```python
from build123d import *

# Parameters (mm, degrees)
REVOLVE_1_ANGLE = 359


with BuildPart() as part:
    # 草图2 → 旋转1 (revolve)
    with BuildSketch(Plane(origin=(0, 0, 0), x_dir=(0, 1, 0), z_dir=(-1, 0, 0))):
        Polygon((37, 0), (41, 0), (41, 0.5), (40.5, 0.5), (40.5, 1), (38.5, 1), (38.5, 2), (40.5, 2), (40.5, 2.5), (41, 2.5), (41, 3), (37, 3), align=None)
    revolve(axis=Axis((0, 0, 0), (0, 0, -1)), revolution_arc=REVOLVE_1_ANGLE)


solid = part.part
```
Geometry check sheet. Reference: the model listing, model coordinates, mm. A direction names the side the tool comes from. Give positions to 0.01 mm unless a question says otherwise; leave off trailing zeros. Loops run counter-clockwise (first coordinate to the right, second up) from the corner with the lowest first, then second, coordinate; pieces in that order, holes last. Notation, with made-up numbers: M 50,56.25 L 59,56.25 A10 cw 59,71.25 Z; hole C 49,34.5 d2. An arc over 180 degrees is marked long. Write item = value, one per line.
(1) Sectioned sample at A-A, the plane y = 0. Record the cut outline in (x, z).
Answer below:
outline = M -41,-3 L -37,-3 L -37,0 L -41,0 L -41,-0.5 L -40.5,-0.5 L -40.5,-1 L -38.5,-1 L -38.5,-2 L -40.5,-2 L -40.5,-2.5 L -41,-2.5 Z; M 37,-3 L 41,-3 L 41,-2.5 L 40.5,-2.5 L 40.5,-2 L 38.5,-2 L 38.5,-1 L 40.5,-1 L 40.5,-0.5 L 41,-0.5 L 41,0 L 37,0 Z
(2) Gauge pin test, flat ends, axial feed: pin 1 Ø24.5 at (x, y) = (-11.5, 19.5) entering from +Z; pin 2 Ø1.5 at (y, z) = (21.5, -0.5) entering from +X. Record the tip position at first contact, or that the pin passes through.
Answer below:
pin_1 = through
pin_2 = 35.36
(3) Release check for a two-part mould opening along X. For faces 4 (the face through (9.3, 39.7, -2.5)), 5 (the face through (1.94, -36.95, -1.48)), 6 (the face through (2.129, -40.444, -0.754)) record: released by +X, released by -X, zero draft, split by the parting line, or undercut.
Answer below:
face_4 = zero draft
face_5 = undercut
face_6 = split by the parting line
(4) Tool access check on faces 1 (the face through (-15, 36, -1)), 2 (the face through (0, 38, -2)), 3 (the face through (37, 6, 0)). Record the directions out of +Z, -Z, +X, -X, +Y, -Y that give a thin tool (end or side, any length) a straight path to the whole face; none if there is none.
Answer below:
face_1 = none
face_2 = +Z, -Z, +Y
face_3 = +Z, +X, -X, +Y, -Y
(5) Sectioned sample at B-B, the plane x = -21.5. Record the cut outline in (y, z).
Answer below:
outline = M -34.91,-3 L -30.11,-3 L -30.11,0 L -34.91,0 L -34.91,-0.5 L -34.32,-0.5 L -34.32,-1 L -31.94,-1 L -31.94,-2 L -34.32,-2 L -34.32,-2.5 L -34.91,-2.5 Z; M 30.11,-3 L 34.91,-3 L 34.91,-2.5 L 34.32,-2.5 L 34.32,-2 L 31.94,-2 L 31.94,-1 L 34.32,-1 L 34.32,-0.5 L 34.91,-0.5 L 34.91,0 L 30.11,0 Z
(6) Material ranges on line 1 (X direction, y = 0, z = -0.95); line 2 (X direction, y = 1, z = -0.25); line 3 (Y direction, x = -10, z = -2.75), recorded low to high. Write a range as [from, to].
Answer below:
line_1 = [-40.5, -37], [37, 40.5]
line_2 = [-40.99, -36.99], [36.99, 40.99]
line_3 = [-39.76, -35.62], [35.62, 39.76]
